```python
from build123d import *

# Parameters (mm, degrees)
SKETCH1_W                       = 15
SKETCH1_H                       = 15
BOSS_EXTRUDE1_DEPTH             = 3
BOSS_EXTRUDE2_START             = -1.18
SKETCH7_W                       = 8
SKETCH7_H                       = 3
BOSS_EXTRUDE2_DEPTH             = 6.18
CIRPATTERN2_COUNT               = 2
CIRPATTERN2_ANGLE               = 60
CIRPATTERN2_THE_OTHER_WAY_COUNT = 2
CIRPATTERN2_THE_OTHER_WAY_ANGLE = 60
TAP_DRILL_FOR_M3_TAP1_D         = 2.5
BOSS_EXTRUDE4_DEPTH             = 3
CUT_EXTRUDE1_START              = -10
CUT_EXTRUDE1_DEPTH              = 10
FILLET12_R                      = 2
SKETCH22_W                      = 31
SKETCH22_H                      = 3
BOSS_EXTRUDE11_DEPTH            = 4
CIRPATTERN8_COUNT               = 2
CIRPATTERN8_ANGLE               = 60
CIRPATTERN8_THE_OTHER_WAY_COUNT = 2
CIRPATTERN8_THE_OTHER_WAY_ANGLE = 60
CUT_EXTRUDE2_DEPTH              = 15
FILLET13_R                      = 2
BOSS_EXTRUDE12_DEPTH            = 2
CIRPATTERN9_COUNT               = 2
CIRPATTERN9_ANGLE               = 60
CIRPATTERN9_THE_OTHER_WAY_COUNT = 2
CIRPATTERN9_THE_OTHER_WAY_ANGLE = 60
SKETCH25_W                      = 2.5
SKETCH25_H                      = 7.427363245
REVOLVE1_ANGLE                  = 61.68
REVOLVE1_OTHER_WAY_ANGLE        = 61.68
FILLET14_R                      = 1


with BuildPart() as part:
    # Sketch1 → Boss-Extrude1 (new body)
    with BuildSketch(Plane(origin=(0, 0, 0), x_dir=(1, 0, 0), z_dir=(0, 1, 0))):
        Rectangle(SKETCH1_W, SKETCH1_H)
    extrude(amount=BOSS_EXTRUDE1_DEPTH)

    # Sketch7 → Boss-Extrude2 (add)
    with BuildSketch(Plane(origin=(0, 0, -7.5), x_dir=(-1, 0, 0), z_dir=(0, 0, -1)).offset(BOSS_EXTRUDE2_START)):
        with Locations((0, 1.5)):
            Rectangle(SKETCH7_W, SKETCH7_H)
    boss_extrude2 = extrude(amount=BOSS_EXTRUDE2_DEPTH)

    # CirPattern2: Boss-Extrude2 ×2 about axis
    cirpattern2_axis = Axis((0, 0, 0), (0, -1, 0))
    for i in range(1, CIRPATTERN2_COUNT):
        add(boss_extrude2.rotate(cirpattern2_axis, i * CIRPATTERN2_ANGLE / (CIRPATTERN2_COUNT - 1)))

    # CirPattern2 the other way: Boss-Extrude2 ×2 about axis
    cirpattern2_the_other_way_axis = Axis((0, 0, 0), (0, 1, 0))
    for i in range(1, CIRPATTERN2_THE_OTHER_WAY_COUNT):
        add(boss_extrude2.rotate(cirpattern2_the_other_way_axis, i * CIRPATTERN2_THE_OTHER_WAY_ANGLE / (CIRPATTERN2_THE_OTHER_WAY_COUNT - 1)))

    # Tap Drill for M3 Tap1 (through all)
    with Locations(Plane(origin=(0, 3, 0), x_dir=(1, 0, 0), z_dir=(0, 1, 0))):
        with Locations((-3.75, -3.75), (-3.75, 3.75), (3.75, -3.75), (3.75, 3.75)):
            Hole(TAP_DRILL_FOR_M3_TAP1_D / 2)

    # Sketch10 → Boss-Extrude4 (add)
    with BuildSketch(Plane(origin=(0, 3, 0), x_dir=(1, 0, 0), z_dir=(0, 1, 0))):
        with BuildLine():
            Line((4.990381057, 7.5), (8.256095748, 9.385461256))
            ThreePointArc((8.256095748, 9.385461256), (6.25, 10.825317547), (4, 11.842719282))
            Line((4, 11.842719282), (4, 7.5))
            Line((4, 7.5), (4.990381057, 7.5))
        make_face()
        with BuildLine():
            ThreePointArc((-4, 11.842719282), (-6.25, 10.825317547), (-8.256095748, 9.385461256))
            Line((-8.256095748, 9.385461256), (-4.990381057, 7.5))
            Line((-4.990381057, 7.5), (-4, 7.5))
            Line((-4, 7.5), (-4, 11.842719282))
        make_face()
    extrude(amount=-BOSS_EXTRUDE4_DEPTH)

    # Sketch21 → Cut-Extrude1 (cut)
    with BuildSketch(Plane(origin=(0, 3, 0), x_dir=(1, 0, 0), z_dir=(0, 1, 0)).offset(CUT_EXTRUDE1_START)):
        with BuildLine():
            ThreePointArc((-4.633883476, 2.866116524), (-4.633883476, 4.633883476), (-2.866116524, 4.633883476))
            Line((-2.866116524, 4.633883476), (-3.396446609, 5.164213562))
            Line((-3.396446609, 5.164213562), (-3.75, 5.517766953))
            ThreePointArc((-3.75, 5.517766953), (-5.517766953, 5.517766953), (-5.517766953, 3.75))
            Line((-5.517766953, 3.75), (-4.633883476, 2.866116524))
        make_face()
        with BuildLine():
            ThreePointArc((-0.5, 2.193741097), (-1.590990258, 1.590990258), (-2.193741097, 0.5))
            Line((-2.193741097, 0.5), (-5.164213562, 0.5))
            ThreePointArc((-5.164213562, 0.5), (-5.664213562, 0), (-5.164213562, -0.5))
            Line((-5.164213562, -0.5), (-2.193741097, -0.5))
            ThreePointArc((-2.193741097, -0.5), (-1.590990258, -1.590990258), (-0.5, -2.193741097))
            Line((-0.5, -2.193741097), (-0.5, -5.164213562))
            ThreePointArc((-0.5, -5.164213562), (0, -5.664213562), (0.5, -5.164213562))
            Line((0.5, -5.164213562), (0.5, -2.193741097))
            ThreePointArc((0.5, -2.193741097), (1.590990258, -1.590990258), (2.193741097, -0.5))
            Line((2.193741097, -0.5), (5.164213562, -0.5))
            ThreePointArc((5.164213562, -0.5), (5.664213562, 0), (5.164213562, 0.5))
            Line((5.164213562, 0.5), (2.193741097, 0.5))
            ThreePointArc((2.193741097, 0.5), (1.590990258, 1.590990258), (0.5, 2.193741097))
            Line((0.5, 2.193741097), (0.5, 5.164213562))
            ThreePointArc((0.5, 5.164213562), (0, 5.664213562), (-0.5, 5.164213562))
            Line((-0.5, 5.164213562), (-0.5, 2.193741097))
        make_face()
        with BuildLine():
            Line((3.75, 5.517766953), (3.396446609, 5.164213562))
            Line((3.396446609, 5.164213562), (2.866116524, 4.633883476))
            ThreePointArc((2.866116524, 4.633883476), (4.633883476, 4.633883476), (4.633883476, 2.866116524))
            Line((4.633883476, 2.866116524), (5.517766953, 3.75))
            ThreePointArc((5.517766953, 3.75), (5.517766953, 5.517766953), (3.75, 5.517766953))
        make_face()
        with BuildLine():
            Line((5.517766953, -3.75), (4.633883476, -2.866116524))
            ThreePointArc((4.633883476, -2.866116524), (4.633883476, -4.633883476), (2.866116524, -4.633883476))
            Line((2.866116524, -4.633883476), (3.75, -5.517766953))
            ThreePointArc((3.75, -5.517766953), (5.517766953, -5.517766953), (5.517766953, -3.75))
        make_face()
        with BuildLine():
            Line((-4.633883476, -2.866116524), (-5.517766953, -3.75))
            ThreePointArc((-5.517766953, -3.75), (-5.517766953, -5.517766953), (-3.75, -5.517766953))
            Line((-3.75, -5.517766953), (-2.866116524, -4.633883476))
            ThreePointArc((-2.866116524, -4.633883476), (-4.633883476, -4.633883476), (-4.633883476, -2.866116524))
        make_face()
    extrude(amount=CUT_EXTRUDE1_DEPTH, mode=Mode.SUBTRACT)

    # Fillet12
    fillet12_edges = [part.edges().sort_by_distance(p)[0] for p in [
        (7.5, 1.5, 7.5),
        (-7.5, 1.5, 7.5),
    ]]
    fillet(fillet12_edges, radius=FILLET12_R)

    # Sketch22 → Boss-Extrude11 (add, symmetric)
    with BuildSketch(Plane(origin=(0, 0, 0), x_dir=(0, 0, -1), z_dir=(1, 0, 0))):
        with Locations((28, 1.5)):
            Rectangle(SKETCH22_W, SKETCH22_H)
    boss_extrude11 = extrude(amount=BOSS_EXTRUDE11_DEPTH, both=True)

    # CirPattern8: Boss-Extrude11 ×2 about axis
    cirpattern8_axis = Axis((0, 0, 0), (0, 1, 0))
    for i in range(1, CIRPATTERN8_COUNT):
        add(boss_extrude11.rotate(cirpattern8_axis, i * CIRPATTERN8_ANGLE / (CIRPATTERN8_COUNT - 1)))

    # CirPattern8 the other way: Boss-Extrude11 ×2 about axis
    cirpattern8_the_other_way_axis = Axis((0, 0, 0), (0, -1, 0))
    for i in range(1, CIRPATTERN8_THE_OTHER_WAY_COUNT):
        add(boss_extrude11.rotate(cirpattern8_the_other_way_axis, i * CIRPATTERN8_THE_OTHER_WAY_ANGLE / (CIRPATTERN8_THE_OTHER_WAY_COUNT - 1)))

    # Sketch23 → Cut-Extrude2 (cut)
    with BuildSketch(Plane(origin=(0, 3, 0), x_dir=(1, 0, 0), z_dir=(0, 1, 0))):
        with BuildLine():
            Line((0, 11.842719282), (2, 11.842719282))
            Line((2, 11.842719282), (1, 32.898140757))
            ThreePointArc((1, 32.898140757), (0, 33.898140757), (-1, 32.898140757))
            Line((-1, 32.898140757), (-2, 11.842719282))
            Line((-2, 11.842719282), (0, 11.842719282))
        make_face()
        Polygon((2, 43.5), (4, 11.842719282), (4, 43.5), align=None)
        Polygon((35.672105065, 25.214101615), (8.256095748, 9.385461256), (36.672105065, 23.482050808), align=None)
        Polygon((-4, 43.5), (-4, 11.842719282), (-2, 43.5), align=None)
        with BuildLine():
            Line((27.990625633, 17.315095782), (9.256095748, 7.653410449))
            Line((9.256095748, 7.653410449), (11.256095748, 4.189308834))
            Line((11.256095748, 4.189308834), (28.990625633, 15.583044975))
            ThreePointArc((28.990625633, 15.583044975), (29.356651037, 16.949070379), (27.990625633, 17.315095782))
        make_face()
        Polygon((-36.672105065, 23.482050808), (-8.256095748, 9.385461256), (-35.672105065, 25.214101615), align=None)
        Polygon((39.672105065, 18.285898385), (38.672105065, 20.017949192), (12.256095748, 2.457258026), align=None)
        with BuildLine():
            Line((-11.256095748, 4.189308834), (-9.256095748, 7.653410449))
            Line((-9.256095748, 7.653410449), (-27.990625633, 17.315095782))
            ThreePointArc((-27.990625633, 17.315095782), (-29.356651037, 16.949070379), (-28.990625633, 15.583044975))
            Line((-28.990625633, 15.583044975), (-11.256095748, 4.189308834))
        make_face()
        Polygon((-12.256095748, 2.457258026), (-38.672105065, 20.017949192), (-39.672105065, 18.285898385), align=None)
    extrude(amount=-CUT_EXTRUDE2_DEPTH, mode=Mode.SUBTRACT)

    # Fillet13
    fillet13_edges = [part.edges().sort_by_distance(p)[0] for p in [
        (4, 1.5, -11.842719282),
        (8.256095748, 1.5, -9.385461256),
        (12.256095748, 1.5, -2.457258026),
        (-12.256095748, 1.5, -2.457258026),
        (7.5, 1.5, 0.288675135),
        (-7.5, 1.5, 0.288675135),
        (-8.256095748, 1.5, -9.385461256),
        (-4, 1.5, -11.842719282),
    ]]
    fillet(fillet13_edges, radius=FILLET13_R)

    # Sketch24 → Boss-Extrude12 (add, symmetric)
    with BuildSketch(Plane(origin=(0, 0, 0), x_dir=(0, 0, -1), z_dir=(1, 0, 0))):
        Polygon((68.233351235, 25), (68.233351235, 17.572636755), (63.498764769, 6.849530075), (45.233351235, 0), (43.5, 0), (43.5, 3), (61.5, 9.75), align=None)
    boss_extrude12 = extrude(amount=BOSS_EXTRUDE12_DEPTH, both=True)

    # CirPattern9: Boss-Extrude12 ×2 about axis
    cirpattern9_axis = Axis((0, 0, 0), (0, 1, 0))
    for i in range(1, CIRPATTERN9_COUNT):
        add(boss_extrude12.rotate(cirpattern9_axis, i * CIRPATTERN9_ANGLE / (CIRPATTERN9_COUNT - 1)))

    # CirPattern9 the other way: Boss-Extrude12 ×2 about axis
    cirpattern9_the_other_way_axis = Axis((0, 0, 0), (0, -1, 0))
    for i in range(1, CIRPATTERN9_THE_OTHER_WAY_COUNT):
        add(boss_extrude12.rotate(cirpattern9_the_other_way_axis, i * CIRPATTERN9_THE_OTHER_WAY_ANGLE / (CIRPATTERN9_THE_OTHER_WAY_COUNT - 1)))

    # Sketch25 → Revolve1 (revolve)
    with BuildSketch(Plane(origin=(0, 0, 0), x_dir=(0, 0, -1), z_dir=(1, 0, 0))):
        with Locations((69.483351235, 21.286318378)):
            Rectangle(SKETCH25_W, SKETCH25_H)
    revolve(axis=Axis((0, 0, 0), (0, 1, 0)), revolution_arc=REVOLVE1_ANGLE)

    # Sketch25 → Revolve1 other way (revolve)
    with BuildSketch(Plane(origin=(0, 0, 0), x_dir=(0, 0, -1), z_dir=(1, 0, 0))):
        with Locations((69.483351235, 21.286318378)):
            Rectangle(SKETCH25_W, SKETCH25_H)
    revolve(axis=Axis((0, 0, 0), (0, -1, 0)), revolution_arc=REVOLVE1_OTHER_WAY_ANGLE)

    # Fillet14
    fillet14_edges = [part.edges().sort_by_distance(p)[0] for p in [
        (-62.267404585, 21.286318378, -33.555585275),
        (62.267404585, 21.286318378, -33.555585275),
    ]]
    fillet(fillet14_edges, radius=FILLET14_R)


solid = part.part
```
The listing builds one solid part. Answer for the finished solid, in the listing's coordinates (mm). A direction names the side the tool comes from. Coordinates: 2 decimals unless noted, no trailing zeros. Write each loop counter-clockwise with the first axis right and the second up, starting at its lowest first coordinate (ties: lowest second). Pieces come first, ordered by that corner, then holes. Notation, with made-up numbers: (87.5, -30.75) -> (116.5, -30.75) arc R17 cw to (116.5, -26.75) -> close; hole circle Ø2 at (-18.75, 33). An arc over 180 degrees is marked (long way). Write each question's results on one line, items separated by ' | '. Start each with the question number.
1) For a pull along X with two mould halves and no side action, classify faces 4 (the flat face through (-23.2, 1.5, -16.8)), 5 (the flat face through (-47.179, 3.473, -27.271)), 6 (the flat face through (3, 0, -11)) as +X half, -X half, draft (parallel to the pull), parting line (faces both ways), or undercut.
2) Flat-ended cylindrical pins translate along their axes: pin 1 Ø15.5 at (x, z) = (19, -16.5) entering from +Y; pin 2 Ø1.5 at (y, z) = (5, -9) entering from +X; pin 3 Ø3.5 at (y, z) = (2, 4) entering from -X; pin 4 Ø3.5 at (y, z) = (1, 2.5) entering from -X. Find the tip coordinate at first contact, or state that the pin passes through.
3) A cutting plane is placed at B-B (z = -48.5). Determine the outline of the cut face in (x, y) (3 decimals), then the cut area to 3 significant figures.
4) A cutting plane is placed at A-A (x = -43). Determine the outline of the cut face in (y, z), then the cut area to 3 significant figures.
5) Straight lines are drawn through the part: probe 1 along Z at (x, y) = (-13, 2); probe 2 along Z at (x, y) = (35, 2.5); probe 3 along Z at (x, y) = (22, 21.75). For each, find the intervals that lie inside material, in ascending order.
6) A tool of negligible diameter and unlimited length cuts with its end or side. For faces 1 (the flat face through (0.5, 1, -4)), 2 (the flat face through (45.371, 6.328, -26.163)), 3 (the cylindrical face through (6.266, 1.521, -10.816)), from which of +Z, -Z, +X, -X, +Y, -Y can it reach the whole face along a straight path? Write none if from no direction.
Values follow:
1) face 4: undercut | face 5: -X half | face 6: draft
2) pin 1: y = 3 | pin 2: through | pin 3: x = -7.5 | pin 4: x = -7.62
3) outline: (-51.487, 17.573) -> (-47.995, 17.573) -> (-47.995, 25) -> (-51.487, 25) -> close; (-2, 1.225) -> (2, 1.225) -> (2, 4.875) -> (-2, 4.875) -> close; (47.995, 17.573) -> (51.487, 17.573) -> (51.487, 25) -> (47.995, 25) -> close | area: 66.5 mm²
4) outline: (1.22, -22.52) -> (2.09, -27.14) -> (5.74, -27.14) -> (4.87, -22.52) -> close; (17.57, -56.16) -> (25, -56.16) -> (25, -52.98) -> (17.57, -52.98) -> close | area: 40.5 mm²
5) probe 1: -11.74 to -9.58, -5.31 to -2.95 | probe 2: -22.65 to -17.58 | probe 3: -67.23 to -64.59
6) face 1: +Y, -Y | face 2: +Z, +Y | face 3: -Z, +Y, -Y
